For this review, take the finished solid that the model builds, in its own axes (mm). A direction names the side the tool comes from. Coordinates: 2 decimals unless noted, no trailing zeros. Loops run counter-clockwise (first coordinate to the right, second up) from the corner with the lowest first, then second, coordinate; pieces in that order, holes last. Notation, with made-up numbers: (65, -19.75) -> (121, -19.75) arc R30 ccw to (121, 16.25) -> close; hole circle Ø1 at (-13.75, 74). An arc over 180 degrees is marked (long way). Answer in a Markdown table with one row per item.
from build123d import *

# Parameters (mm, degrees)
BOSS_EXTRUDE1_DEPTH = 420
BOSS_EXTRUDE2_DEPTH = 10


with BuildPart() as part:
    # Sketch1 → Boss-Extrude1 (new body)
    with BuildSketch(Plane(origin=(0, 0, 0), x_dir=(1, 0, 0), z_dir=(0, 1, 0))):
        Polygon((-113.787540309, 45.905289316), (-233.518909136, 165.636658142), (-165.636658142, 233.518909136), (-45.905289316, 113.787540309), (44.422091789, 113.787540309), (164.153460615, 233.518909136), (232.035711609, 165.636658142), (112.304342783, 45.905289316), (112.304342783, -44.422091789), (232.035711609, -164.153460615), (164.153460615, -232.035711609), (44.422091789, -112.304342783), (-45.905289316, -112.304342783), (-165.636658142, -232.035711609), (-233.518909136, -164.153460615), (-113.787540309, -44.422091789), align=None)
        Polygon((-50.047424939, -102.304342783), (48.564227412, -102.304342783), (164.153460615, -217.893575985), (217.893575985, -164.153460615), (102.304342783, -48.564227412), (102.304342783, 50.047424939), (217.893575985, 165.636658142), (164.153460615, 219.376773512), (48.564227412, 103.787540309), (-50.047424939, 103.787540309), (-165.636658142, 219.376773512), (-219.376773512, 165.636658142), (-103.787540309, 50.047424939), (-103.787540309, -48.564227412), (-219.376773512, -164.153460615), (-165.636658142, -217.893575985), align=None, mode=Mode.SUBTRACT)
    extrude(amount=-BOSS_EXTRUDE1_DEPTH)

    # Sketch3 → Boss-Extrude2 (add)
    with BuildSketch(Plane.XZ.offset(420)):
        Polygon((-113.787540309, 44.422091789), (-113.787540309, -45.905289316), (-233.518909136, -165.636658142), (-165.636658142, -233.518909136), (-45.905289316, -113.787540309), (44.422091789, -113.787540309), (164.153460615, -233.518909136), (232.035711609, -165.636658142), (112.304342783, -45.905289316), (112.304342783, 44.422091789), (232.035711609, 164.153460615), (164.153460615, 232.035711609), (44.422091789, 112.304342783), (-45.905289316, 112.304342783), (-165.636658142, 232.035711609), (-233.518909136, 164.153460615), align=None)
    extrude(amount=BOSS_EXTRUDE2_DEPTH)


solid = part.part
Item 1: Take a section at C-C, the plane x = 37. State the section outline as (y, z) points, and give its area (3 significant figures).
Worked answers:
| item | result |
|---|---|
| outline | (-430, -113.79) -> (0, -113.79) -> (0, -103.79) -> (-420, -103.79) -> (-420, 102.3) -> (0, 102.3) -> (0, 112.3) -> (-430, 112.3) -> close |
| area | 10,700 mm² |
Item 2: For faces 4 (the flat face through (-103.788, -207, -1)), 5 (the flat face through (173, -212, -106.6)), 6 (the flat face through (-174.491, -211.99, 105.126)), 7 (the flat face through (198.57, -211.99, 197.62)), 8 (the flat face through (0, -212, 112.304)), list the 3-axis set-ups (+Z, -Z, +X, -X, +Y, -Y) from which the entire face can be reached by the end or side of a thin tool; tool diameter is ignored.
Worked answers:
| item | result |
|---|---|
| face 4 | +Y |
| face 5 | +X, +Y, -Y |
| face 6 | -X, +Y, -Y |
| face 7 | +Z, +X, +Y, -Y |
| face 8 | +Z, +Y, -Y |
Item 3: The part is to be moulded in two halves that separate along Z. For faces 1 (the flat face through (112.304, -212, -1)), 2 (the flat face through (-200.053, -211.99, -199.103)), 3 (the flat face through (-104.9, -212, 171.3)), say which applies: +Z half, -Z half, draft (parallel to the pull), parting line (faces both ways), or undercut.
Worked answers:
| item | result |
|---|---|
| face 1 | undercut |
| face 2 | -Z half |
| face 3 | +Z half |
Item 4: Take a section at B-B, the plane z = 173. State the section outline as (x, y) points.
Worked answers:
| item | result |
|---|---|
| outline | (-224.67, -430) -> (-106.6, -430) -> (-106.6, 0) -> (-120.74, 0) -> (-120.74, -420) -> (-210.53, -420) -> (-210.53, 0) -> (-224.67, 0) -> close; (105.12, -430) -> (223.19, -430) -> (223.19, 0) -> (209.05, 0) -> (209.05, -420) -> (119.26, -420) -> (119.26, 0) -> (105.12, 0) -> close |
Item 5: Take a section at D-D, the plane x = 204. State the section outline as (y, z) points, and give its area (3 significant figures).
Worked answers:
| item | result |
|---|---|
| outline | (-430, -193.67) -> (0, -193.67) -> (0, -179.53) -> (-420, -179.53) -> (-420, -151.74) -> (0, -151.74) -> (0, -137.6) -> (-430, -137.6) -> close; (-430, 136.12) -> (0, 136.12) -> (0, 150.26) -> (-420, 150.26) -> (-420, 178.05) -> (0, 178.05) -> (0, 192.19) -> (-430, 192.19) -> close |
| area | 24,900 mm² |
Item 6: Insertion check: pin 1 (4 mm diameter, centred on y = -241.5, z = -66, fed in from -X); pin 2 (1 mm diameter, centred on y = -63.5, z = -23, fed in from -X); pin 3 (2 mm diameter, centred on y = -76.5, z = 5, fed in from +X). Each pin has a flat end and moves straight along its axis. Give the tip position at first contact, or say it passes through.
Worked answers:
| item | result |
|---|---|
| pin 1 | x = -135.88 |
| pin 2 | x = -113.79 |
| pin 3 | x = 112.3 |
Item 7: For L1, parallel to X at y = -62, z = -9.5; L2, parallel to X at y = -140.5, z = -135.5; L3, parallel to X at y = -130, z = -196, list the stretches that pass through material, from the lowest coordinate up.
Worked answers:
| item | result |
|---|---|
| L1 | -113.79 to -103.79, 102.3 to 112.3 |
| L2 | -203.38 to -189.24, -81.76 to -67.62, 66.13 to 80.28, 187.76 to 201.9 |
| L3 | -203.16 to -189.01, -142.26 to -128.12, 126.63 to 140.78, 187.53 to 201.67 |
